Can you work these out from the model? Positions are in its coordinate system, mm. A direction names the side the tool comes from. Round coordinates to 2 decimals unless told otherwise and drop trailing zeros. Write each loop counter-clockwise with the first axis right and the second up, starting at its lowest first coordinate (ties: lowest second). Pieces come first, ordered by that corner, then holes. Notation, with made-up numbers: (71.25, 69.25) - (119.25, 69.25) arc R29 ccw to (119.25, 90.25) - close; hole circle Ø8 at (-39, 27). An arc over 180 degrees is marked (long way). One line per item, written item: value. Start each with the question number.
(1) On a 3-axis mill with a long thin cutter (end or side, diameter ignored), from which of +Z, -Z, +X, -X, +Y, -Y can I reach the whole of each face in a straight line? I mean faces 1 (the face through (137.9, 39.4, 81.1)), 2 (the face through (-109, 39, -239.976)), 3 (the face through (1, 359, -366.676)), 4 (the face through (1, 39, -159.976)). Say none if no direction works.
(2) If I drill on L1, parallel to X at y = 36, z = 121; L2, parallel to X at y = 255, z = -418.5; L3, parallel to X at y = 349.5, z = -387.5, over which ranges is the centre line in solid material (lowest first)? Write a range as from..to.
(3) I want a section at D-D on z = -191.5. List the corners of the cut face in (x, y) for me.
(4) I'm going to push flat-ended pins straight in: pin 1 Ø18 at (x, z) = (15.5, -83.5) entering from -Y; pin 2 Ø17.5 at (x, y) = (-99, 43.5) entering from -Z; pin 3 Ø3 at (x, z) = (0.5, -304.5) entering from +Y. Where does each tip first touch, or does it pass through?
(5) I want a section at B-B on z = 94.5. List the corners of the cut face in (x, y) for me.
(6) Thinking about a two-plate mould opening in Y: for faces 5 (the face through (-40, 603, -142)), 6 (the face through (1.12, 129.12, -351.74)), 7 (the face through (0.56, 450.761, 73.295)), 8 (the face through (1, 673.4, -148)), which applies, +Y half, -Y half, draft (parallel to the pull), parting line (faces both ways), or undercut?
(7) I want a section at A-A on x = 22. List the corners of the cut face in (y, z) for me.
(8) I want a section at C-C on y = 374.5. List the corners of the cut face in (x, z) for me, plus the area to 3 significant figures.
from build123d import *

# Parameters (mm, degrees)
SALIENTE_EXTRUIR1_DEPTH = 80
SALIENTE_EXTRUIR2_DEPTH = 80
SALIENTE_EXTRUIR4_DEPTH = 40


with BuildPart() as part:
    # Croquis1 → Saliente-Extruir1 (new body)
    with BuildSketch(Plane(origin=(0, 0, 0), x_dir=(1, 0, 0), z_dir=(0, 1, 0))):
        Polygon((-138.55, 239.975639389), (-277.1, 0), (-138.55, -239.975639389), (138.55, -239.975639389), (277.1, 0), (138.55, 239.975639389), align=None)
        Polygon((-92.361978465, 159.975639389), (-184.72395693, 0), (-92.361978465, -159.975639389), (92.361978465, -159.975639389), (184.72395693, 0), (92.361978465, 159.975639389), align=None, mode=Mode.SUBTRACT)
    extrude(amount=SALIENTE_EXTRUIR1_DEPTH)

    # Croquis2 → Saliente-Extruir2 (add, symmetric)
    with BuildSketch(Plane(origin=(0, 0, 0), x_dir=(0, 0, -1), z_dir=(1, 0, 0))):
        Polygon((239.975639389, 0), (466.675639389, 261.9), (326.675639389, 261.9), (169.223443894, 80), (169.223443894, 0), align=None)
    extrude(amount=SALIENTE_EXTRUIR2_DEPTH, both=True)

    # Croquis3 → Saliente-Extruir4 (add, symmetric)
    with BuildSketch(Plane(origin=(0, 0, 0), x_dir=(0, 0, -1), z_dir=(1, 0, 0))):
        with BuildLine():
            Line((366.675639389, 453.4), (366.675639389, 261.9))
            Line((366.675639389, 261.9), (466.675639389, 261.9))
            Line((466.675639389, 261.9), (466.675639389, 453.4))
            ThreePointArc((466.675639389, 453.4), (402.23913125, 608.963491861), (246.675639389, 673.4))
            Line((246.675639389, 673.4), (46.675639389, 673.4))
            ThreePointArc((46.675639389, 673.4), (-173.324360611, 453.4), (46.675639389, 233.4))
            Line((46.675639389, 233.4), (106.675639389, 233.4))
            Line((106.675639389, 233.4), (106.675639389, 333.4))
            Line((106.675639389, 333.4), (46.675639389, 333.4))
            ThreePointArc((46.675639389, 333.4), (-73.324360611, 453.4), (46.675639389, 573.4))
            Line((46.675639389, 573.4), (246.675639389, 573.4))
            ThreePointArc((246.675639389, 573.4), (331.528453131, 538.252813742), (366.675639389, 453.4))
        make_face()
    extrude(amount=SALIENTE_EXTRUIR4_DEPTH, both=True)


solid = part.part
Established:
1. face 1: +Y, -Y
1. face 2: -Z, -X, +Y, -Y
1. face 3: +X, -X
1. face 4: -Y
2. L1: -207.24..-114.86, 114.86..207.24
2. L2: -80..80
2. L3: -40..40
3. outline: (-166.54, 0) - (166.54, 0) - (166.54, 80) - (80, 80) - (80, 105.74) - (-80, 105.74) - (-80, 80) - (-166.54, 80) - close; (-40, 573.4) - (40, 573.4) - (40, 673.4) - (-40, 673.4) - close
4. pin 1: y = 233.4
4. pin 2: z = -239.98
4. pin 3: y = 666.07
5. outline: (-222.54, 0) - (-130.16, 0) - (-130.16, 80) - (-222.54, 80) - close; (-40, 284.67) - (40, 284.67) - (40, 622.13) - (-40, 622.13) - close; (130.16, 0) - (222.54, 0) - (222.54, 80) - (130.16, 80) - close
6. face 5: draft
6. face 6: -Y half
6. face 7: undercut
6. face 8: +Y half
7. outline: (0, -239.98) - (261.9, -466.68) - (453.4, -466.68) arc R220 ccw to (673.4, -246.68) - (673.4, -46.68) arc R220 ccw to (233.4, -46.68) - (233.4, -106.68) - (333.4, -106.68) - (333.4, -46.68) arc R120 cw to (573.4, -46.68) - (573.4, -246.68) arc R120 cw to (453.4, -366.68) - (261.9, -366.68) - (261.9, -326.68) - (80, -169.22) - (80, -159.98) - (0, -159.98) - close; (0, 159.98) - (80, 159.98) - (80, 239.98) - (0, 239.98) - close
8. outline: (-40, -466.68) - (40, -466.68) - (40, -366.68) - (-40, -366.68) - close; (-40, 43.74) - (40, 43.74) - (40, 158.69) - (-40, 158.69) - close
8. area: 17,200 mm2
